The model under review builds one solid part; all positions refer to its coordinate system, in mm. Round coordinates to 2 decimals unless told otherwise and drop trailing zeros. Write each loop counter-clockwise with the first axis right and the second up, starting at its lowest first coordinate (ties: lowest second). Pieces come first, ordered by that corner, then holes. Notation, with made-up numbers: (51.25, -31.75) -> (80.25, -31.75) arc R30 ccw to (80.25, 1.25) -> close; hole circle Ø8 at (21, 42.25). An arc over 180 degrees is marked (long way). Answer as a JSON object with one key per item and string values. Group by question number.
1) We need section A-A, the plane z = 16. Write out the cut boundary in (x, y).
2) We need section B-B, the plane x = -19. Write out the cut boundary in (y, z), then the cut area to 3 significant figures.
3) To check wall thickness, follow probe 1 along X at (y, z) = (2.85, -40); probe 2 along Z at (x, y) = (0, 2.6); probe 3 along X at (y, z) = (4.75, -0.5). State the ranges of each line that lie inside material, in increasing order. Write a range as [from, to].
4) We need section C-C, the plane y = 3.95. Write out the cut boundary in (x, z).
from build123d import *

# Parameters (mm, degrees)
SKETCH1_W           = 90
SKETCH1_H           = 90
SKETCH1_R           = 5
BOSS_EXTRUDE1_DEPTH = 5
SKETCH2_R           = 1.5
CUT_EXTRUDE1_DEPTH  = 6
FILLET1_R           = 5


with BuildPart() as part:
    # Sketch1 → Boss-Extrude1 (new body)
    with BuildSketch(Plane(origin=(0, 0, 0), x_dir=(1, 0, 0), z_dir=(0, 1, 0))):
        Rectangle(SKETCH1_W, SKETCH1_H)
        Circle(SKETCH1_R, mode=Mode.SUBTRACT)
        with BuildLine():
            ThreePointArc((-21.213203436, -21.213203436), (21.213203436, -21.213203436), (21.213203436, 21.213203436))
            ThreePointArc((21.213203436, 21.213203436), (14.142135624, 21.213203436), (14.142135624, 14.142135624))
            ThreePointArc((14.142135624, 14.142135624), (14.142135624, -14.142135624), (-14.142135624, -14.142135624))
            ThreePointArc((-14.142135624, -14.142135624), (-21.213203436, -14.142135624), (-21.213203436, -21.213203436))
        make_face(mode=Mode.SUBTRACT)
    extrude(amount=BOSS_EXTRUDE1_DEPTH)

    # Sketch2 → Cut-Extrude1 (cut, through all)
    with BuildSketch(Plane(origin=(0, 5, 0), x_dir=(1, 0, 0), z_dir=(0, 1, 0))):
        with Locations((-40, 40)):
            Circle(SKETCH2_R)
        with Locations((40, 40)):
            Circle(SKETCH2_R)
        with Locations((40, -40)):
            Circle(SKETCH2_R)
        with Locations((-40, -40)):
            Circle(SKETCH2_R)
    extrude(amount=-CUT_EXTRUDE1_DEPTH, mode=Mode.SUBTRACT)

    # Fillet1
    fillet1_edges = [part.edges().sort_by_distance(p)[0] for p in [
        (45, 2.5, 45),
        (-45, 2.5, 45),
        (-45, 2.5, -45),
        (45, 2.5, -45),
    ]]
    fillet(fillet1_edges, radius=FILLET1_R)


solid = part.part
Here are the results:
{
 "1": {"outline": "(-45, 0) -> (-22.39, 0) -> (-22.39, 5) -> (-45, 5) -> close; (-12, 0) -> (12, 0) -> (12, 5) -> (-12, 5) -> close; (25.38, 0) -> (45, 0) -> (45, 5) -> (25.38, 5) -> close"},
 "2": {"outline": "(0, -45) -> (5, -45) -> (5, 12.86) -> (0, 12.86) -> close; (0, 23.22) -> (5, 23.22) -> (5, 45) -> (0, 45) -> close", "area": "398 mm^2"},
 "3": {"probe 1": "x = [-45, -41.5], [-38.5, 38.5], [41.5, 45]", "probe 2": "z = [-45, -5], [5, 20], [30, 45]", "probe 3": "x = [-45, -4.97], [4.97, 19.99], [30, 45]"},
 "4": {"outline": "(-45, -40) arc R5 ccw to (-40, -45) -> (40, -45) arc R5 ccw to (45, -40) -> (45, 40) arc R5 ccw to (40, 45) -> (-40, 45) arc R5 ccw to (-45, 40) -> close; hole circle Ø3 at (-40, -40); hole circle Ø3 at (-40, 40); hole (-21.21, 21.21) arc R5 ccw to (-14.14, 14.14) arc R20 cw to (14.14, -14.14) arc R5 ccw to (21.21, -21.21) arc R30 ccw to start; hole circle Ø10 at (0, 0); hole circle Ø3 at (40, -40); hole circle Ø3 at (40, 40)"}
}
